Autodesk Inventor part; units mm, degrees
ref_plane "Work Plane1" through (12, 0, 0) normal (1, 0, 0) x (0, 1, 0)
ref_plane "Work Plane2" through (12, 0, -10) normal (0.9986, -0.0533, 0) x (0.0533, 0.9986, 0)
ref_plane "YZ Plane" through (0, 0, 0) normal (1, 0, 0) x (0, 1, 0)
sketch "Skizze1" plane through (0, 0, 0) normal (0, 0, 1) x (1, 0, 0)
  line L0 (0, 0) -> (12, 0)
  line L1 (0.5, 2) -> (11.5, 2)
  arc A0 (0.5, 2) -> (0, 0) centre (4.25, 0) ccw
  arc A1 (12, 0) -> (11.5, 2) centre (7.75, 0) ccw
  line L2 (12, 0) -> (12, 1.68) construction
  line L3 (12, 1.68) -> (6, 2) construction
  line L4 (-12.8617, 0) -> (72.8617, 0)
  line L5 (0, 12.1847) -> (0, -2.0308)
  point P0 (6, 0)
  dimension "d0" = 4
  dimension "d1" = 12
  dimension "d2" = 3.36
  dimension "d12" = 6
  dimension "d17" = 0.5
  dimension "d18" = 0.5
revolve "Körper" add sketch "Skizze1" angle 360 about axis through (0, 0, 0) along (1, 0, 0)
ref_plane "Work Plane1" through (12, 0, 0) normal (1, 0, 0) x (0, 1, 0)
sketch "Skizze2" plane through (12, 0, 0) normal (1, 0, 0) x (0, 1, 0)
  line L0 (0, -14) -> (0, 14)
ref_plane "Work Plane2" through (12, 0, -10) normal (0.9986, -0.0533, 0) x (0.0533, 0.9986, 0)
sketch "Skizze3" plane through (12, 0, -10) normal (0.9986, -0.0533, 0) x (0.0533, 0.9986, 0)
  ellipse E0 centre (-0.0266, 10) end of major axis (-0.0266, 12) minor radius 1.9972
  line L0 (-0.3195, 10) -> (1.6776, 10)
  line L1 (1.6776, 10) -> (1.9607, 10.1982)
  line L2 (1.6776, 10) -> (1.9607, 9.8018)
  arc A0 (1.9607, 9.8018) -> (1.9607, 10.1982) centre (-0.0266, 10) ccw
  dimension "d7" = 70
extrude "Nut" cut sketch "Skizze3" against normal up to next contours L2 L1 E0 picked at (1.8688, 9.9009)
pattern_circular "Nuten" count 3 over 360 about axis through (6, 0, 0) along (1, 0, 0) of "Nut"
equation "\"d0\" = NND"
equation "\"d1\" = NLG"
equation "\"d2\" = 0.84 * NND"
equation "\"d18\" = KAH"
equation "\"d8\" = 0.5 * NLG"
equation "\"NND\" = 4"
equation "\"NLG\" = 12"
equation "\"KAH\" = 0.5"
equation "\"d3\" = NLG"
equation "\"d6\" = -d5"
equation "\"FAC\" = 0.5"
equation "\"NND1\" = 4.25"
equation "\"NLG1\" = 11"
properties part number "ISO 8745 - 4 x 12" material "Edelstahl, austenitisch"
Design review of the part built by this model. Coordinates are the model's own, in mm. Coordinates: 2 decimals unless noted, no trailing zeros. Write each loop counter-clockwise with the first axis right and the second up, starting at its lowest first coordinate (ties: lowest second). Pieces come first, ordered by that corner, then holes.
1) Add section C-C (z = 0.55). Write out the cut boundary in (x, y), plus the area to 3 significant figures.
2) Add section B-B (y = 0). Write out the cut boundary in (x, z), plus the area to 3 significant figures.
3) To check wall thickness, follow L1, parallel to X at y = 1.3, z = -0.6; L2, parallel to Z at x = 9.5, y = -1; L3, parallel to Y at x = 4, z = -0.4. State the ranges of each line that lie inside material, in increasing order.
4) Add section D-D (x = 2). Write out the cut boundary in (y, z), plus the area to 3 significant figures.
5) Insertion check: pin 1 (1 mm diameter, centred on x = 5.5, z = -1, fed in from -Y). The pin has a flat end and moves straight along its axis. Give the tip position at first contact, or say it passes through.
Check result:
1. outline: (0.5, -1.92) - (11.5, -1.92) arc R4.21 ccw to (11.5, 1.92) - (0.5, 1.92) arc R4.21 ccw to start
1. area: 44.7 mm2
2. outline: (0.5, -2) - (11.5, -2) arc R4.25 ccw to (11.5, 2) - (0.5, 2) arc R4.25 ccw to start
2. area: 46.7 mm2
3. L1: x = 0.25 to 11.75
3. L2: z = -1.61 to 1.61
3. L3: y = -1.96 to 1.96
4. outline: circle Ø4 at (0, 0)
4. area: 12.6 mm2
5. pin 1: stops at y = -1.94
